Design review of the part built by this model. Coordinates are the model's own, in mm. Face numbers are marked on the shaded views. A direction names the side the tool comes from. Coordinates: 2 decimals unless noted, no trailing zeros. Write each loop counter-clockwise with the first axis right and the second up, starting at its lowest first coordinate (ties: lowest second). Pieces come first, ordered by that corner, then holes.
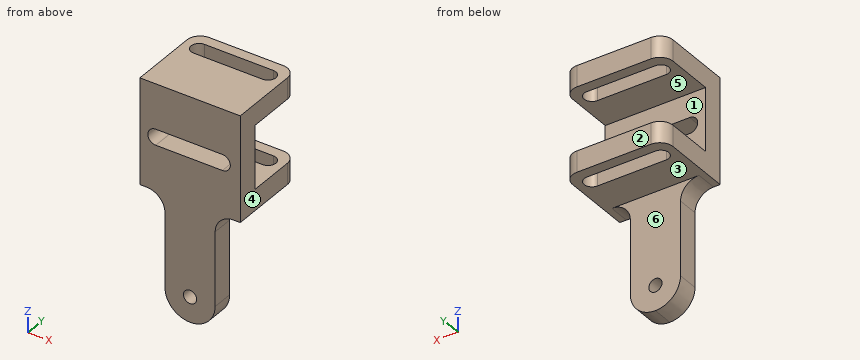
```python
from build123d import *

# Parameters (mm, degrees)
ESTRUSIONE_ESTRUSIONE1_DEPTH = 38
RACCORDO1_R                  = 10
SCHIZZO3_W                   = 38
SCHIZZO3_H                   = 89
ESTRUSIONE_ESTRUSIONE2_DEPTH = 16
RACCORDO3_START              = -1
RACCORDO3_DEPTH              = 18
RACCORDO4_DEPTH              = 16
FORO_10_0_10_1_D             = 10
FORO_10_0_10_1_ON_FACE_2_D   = 10
TAGLIO_ESTRUSIONE1_DEPTH     = 115.93041384
TAGLIO_ESTRUSIONE2_REACH     = 144.13


with BuildPart() as part:
    # Schizzo2 → Estrusione-Estrusione1 (new, symmetric)
    with BuildSketch(Plane(origin=(0, 0, 0), x_dir=(0, 0, -1), z_dir=(1, 0, 0))):
        Polygon((-24, 16), (-24, 62), (-40, 62), (-40, 0), (40, 0), (40, 62), (24, 62), (24, 16), align=None)
    extrude(amount=ESTRUSIONE_ESTRUSIONE1_DEPTH, both=True)

    # Raccordo1
    raccordo1_edges = [part.edges().sort_by_distance(p)[0] for p in [
        (-38, 62, -32),
        (38, 62, -32),
        (38, 62, 32),
        (-38, 62, 32),
    ]]
    fillet(raccordo1_edges, radius=RACCORDO1_R)

    # Schizzo3 → Estrusione-Estrusione2 (add)
    with BuildSketch(Plane.XZ):
        with Locations((0, -84.5)):
            Rectangle(SCHIZZO3_W, SCHIZZO3_H)
    extrude(amount=-ESTRUSIONE_ESTRUSIONE2_DEPTH)

    # Raccordo3: read off the stored shape, not the designer's step
    # Raccordo3 outline → Raccordo3 (cut)
    with BuildSketch(Plane(origin=(0, 0, 0), x_dir=(1, 0, 0), z_dir=(0, 1, 0)).offset(RACCORDO3_START)):
        with BuildLine():
            Line((-19, 129), (-19, 110))
            add(Edge.make_bspline(
                [(-19, 110), (-19, 129), (0, 129)],
                knots=[0, 0, 0, 1, 1, 1], degree=2, weights=[1, 0.707106781, 1]))
            Line((0, 129), (-19, 129))
        make_face()
        with BuildLine():
            Line((19, 129), (0, 129))
            add(Edge.make_bspline(
                [(0, 129), (19, 129), (19, 110)],
                knots=[0, 0, 0, 1, 1, 1], degree=2, weights=[1, 0.707106781, 1]))
            Line((19, 110), (19, 129))
        make_face()
    extrude(amount=RACCORDO3_DEPTH, mode=Mode.SUBTRACT)

    # Raccordo4: read off the stored shape, not the designer's step
    # Raccordo4 outline → Raccordo4 (add)
    with BuildSketch(Plane(origin=(0, 0, 0), x_dir=(1, 0, 0), z_dir=(0, 1, 0))):
        with BuildLine():
            Line((19, 54), (19, 40))
            Line((19, 40), (33, 40))
            add(Edge.make_bspline(
                [(19, 54), (19, 40), (33, 40)],
                knots=[0, 0, 0, 1, 1, 1], degree=2, weights=[1, 0.707106781, 1]))
        make_face()
        with BuildLine():
            add(Edge.make_bspline(
                [(-33, 40), (-19, 40), (-19, 54)],
                knots=[0, 0, 0, 1, 1, 1], degree=2, weights=[1, 0.707106781, 1]))
            Line((-33, 40), (-19, 40))
            Line((-19, 40), (-19, 54))
        make_face()
    extrude(amount=RACCORDO4_DEPTH)

    # Foro Ø10.0 (10)-1 (through all)
    with Locations(Plane(origin=(4.7e-08, 16, -110.000000174), x_dir=(0, 0, 1), z_dir=(0, 1, 0))):
        with Locations((0, 0)):
            Hole(FORO_10_0_10_1_D / 2)

    # Foro Ø10.0 (10)-1 on face 2 (through all)
    with Locations(Plane(origin=(0, 0, -110), x_dir=(0, 0, -1), z_dir=(0, -1, 0))):
        with Locations((0, 0)):
            Hole(FORO_10_0_10_1_ON_FACE_2_D / 2)

    # Schizzo5 → Taglio-Estrusione1 (cut, through all)
    with BuildSketch(Plane(origin=(0, 0, -40), x_dir=(-1, 0, 0), z_dir=(0, 0, -1))):
        with BuildLine():
            Line((-26.051804846, 54), (26.051804846, 54))
            ThreePointArc((26.051804846, 54), (32.051804846, 48), (26.051804846, 42))
            Line((26.051804846, 42), (-26.051804846, 42))
            ThreePointArc((-26.051804846, 42), (-32.051804846, 48), (-26.051804846, 54))
        make_face()
    extrude(amount=-TAGLIO_ESTRUSIONE1_DEPTH, mode=Mode.SUBTRACT)

    # Schizzo6 → Taglio-Estrusione2 (cut, up to next)
    with BuildSketch(Plane(origin=(0, 16, 0), x_dir=(1, 0, 0), z_dir=(0, 1, 0)), mode=Mode.PRIVATE) as taglio_estrusione2_sk1:
        with BuildLine():
            Line((-25.97197238, 6), (24.454717483, 6))
            ThreePointArc((24.454717483, 6), (30.454717483, 0), (24.454717483, -6))
            Line((24.454717483, -6), (-25.97197238, -6))
            ThreePointArc((-25.97197238, -6), (-31.97197238, 0), (-25.97197238, 6))
        make_face()
    taglio_estrusione2_tool1 = extrude(taglio_estrusione2_sk1.sketch, amount=-TAGLIO_ESTRUSIONE2_REACH, mode=Mode.PRIVATE) & part.part
    add(taglio_estrusione2_tool1.solids().sort_by_distance((-0.758627, 16, 0))[0], mode=Mode.SUBTRACT)


solid = part.part
```
(1) Consider section D-D (z = -35.5). Give the boundary of the cut face in (x, y), plus the area to 3 significant figures.
(2) Consider section C-C (y = 39.5). Give the boundary of the cut face in (x, z).
(3) Mouldability with a two-part tool opening along Z and no side actions: class the marked faces 1, 2 and 3 as +Z half, -Z half, draft (parallel to the pull), parting line (faces both ways), or undercut.
(4) Wall thickness on line 1 (Z direction, x = 25.5, y = 30); line 2 (Y direction, x = 16.5, z = -33.5); line 3 (X direction, y = 6, z = -110): over which ranges is each line inside the solid? List them lowest first.
(5) Insertion check: pin 1 Ø5 at (y, z) = (10.5, -73) entering from -X; pin 2 Ø1 at (x, y) = (23, 14.5) entering from -Z; pin 3 Ø17.5 at (y, z) = (6.5, -95.5) entering from +X; pin 4 Ø13 at (x, y) = (4, 8.5) entering from -Z. Each pin has a flat end and moves straight along its axis. Give the tip position at first contact, or say it passes through.
(6) Consider section B-B (y = 48). Give the boundary of the cut face in (x, z), plus the area to 3 significant figures.
(7) For the marked faces 4, 5 and 6, list the 3-axis set-ups (+Z, -Z, +X, -X, +Y, -Y) from which the entire face can be reached by the end or side of a thin tool; tool diameter is ignored.
(8) Consider section A-A (z = 0). Give the boundary of the cut face in (x, y).
Results:
1. outline: (-38, 0) - (38, 0) - (38, 52) arc R10 ccw to (28, 62) - (-28, 62) arc R10 ccw to (-38, 52) - close; hole (-26.05, 42) - (26.05, 42) arc R6 ccw to (26.05, 54) - (-26.05, 54) arc R6 ccw to start
1. area: 3,930 mm2
2. outline: (-38, -40) - (38, -40) - (38, -24) - (-38, -24) - close; (-38, 24) - (38, 24) - (38, 40) - (-38, 40) - close
3. face 1: undercut
3. face 2: draft
3. face 3: -Z half
4. line 1: z = -40 to -24, 24 to 40
4. line 2: y = 0 to 42, 54 to 62
4. line 3: x = -19 to -5, 5 to 19
5. pin 1: stops at x = -19
5. pin 2: stops at z = -44.74
5. pin 3: stops at x = 19
5. pin 4: stops at z = -129
6. outline: (-38, -40) - (-32.05, -40) - (-32.05, -24) - (-38, -24) - close; (-38, 24) - (-32.05, 24) - (-32.05, 40) - (-38, 40) - close; (32.05, -40) - (38, -40) - (38, -24) - (32.05, -24) - close; (32.05, 24) - (38, 24) - (38, 40) - (32.05, 40) - close
6. area: 381 mm2
7. face 4: +Z, -Z, +X, +Y, -Y
7. face 5: +X, -X, +Y
7. face 6: -Z, +X, -X, +Y
8. outline: (-38, 0) - (-31.97, 0) - (-31.97, 16) - (-38, 16) - close; (30.45, 0) - (38, 0) - (38, 16) - (30.45, 16) - close
